Geometry: see drawing. Coordinates: mm, zero at the bounding-box minimum. Coordinates: 2 decimals unless noted, no trailing zeros. Loops run counter-clockwise (first coordinate to the right, second up) from the corner with the lowest first, then second, coordinate; pieces in that order, holes last. Notation, with made-up numbers: (80, 57.5) - (93, 57.5) arc R32 ccw to (93, 83.5) - close; hole circle Ø7 at (-32.5, 49). An arc over 180 degrees is marked (long way). Use a Markdown table: item, result. Add a question column.
1. Section query B-B on z = 2.5. Return the cut outline in (x, y).
2. Ray query, L1, parallel to X at y = 15, z = 3.45; L2, parallel to Z at x = 21, y = 2; L3, parallel to Y at x = 37.5, z = 0.5. Return the intervals inside material, ascending. Write a range as [from, to].
3. Section query D-D on z = 12. Return the cut outline in (x, y).
4. Contact query for flat-ended pins moving along their axis: P1, Ø4, axis at x = 33, y = 19.5, coming from the +Z side; P2, Ø10.5, axis at x = 23.6, y = 15, coming from the -Z side; P3, Ø2, axis at y = 5, z = 2, coming from the -X side; P4, Ø1.5, axis at y = 24, z = 11.5, coming from the +X side. Output: stop coordinate, or through.
5. Draft query along Y for the marked faces 1, 2, 3 and 4. Return one class per face: released by +Y, released by -Y, zero draft, split by the parting line, or undercut.
6. Section query C-C on y = 20.75. Return the cut outline in (x, z).
7. Section query A-A on y = 15. Return the cut outline in (x, z), then the cut area to 3 significant figures.
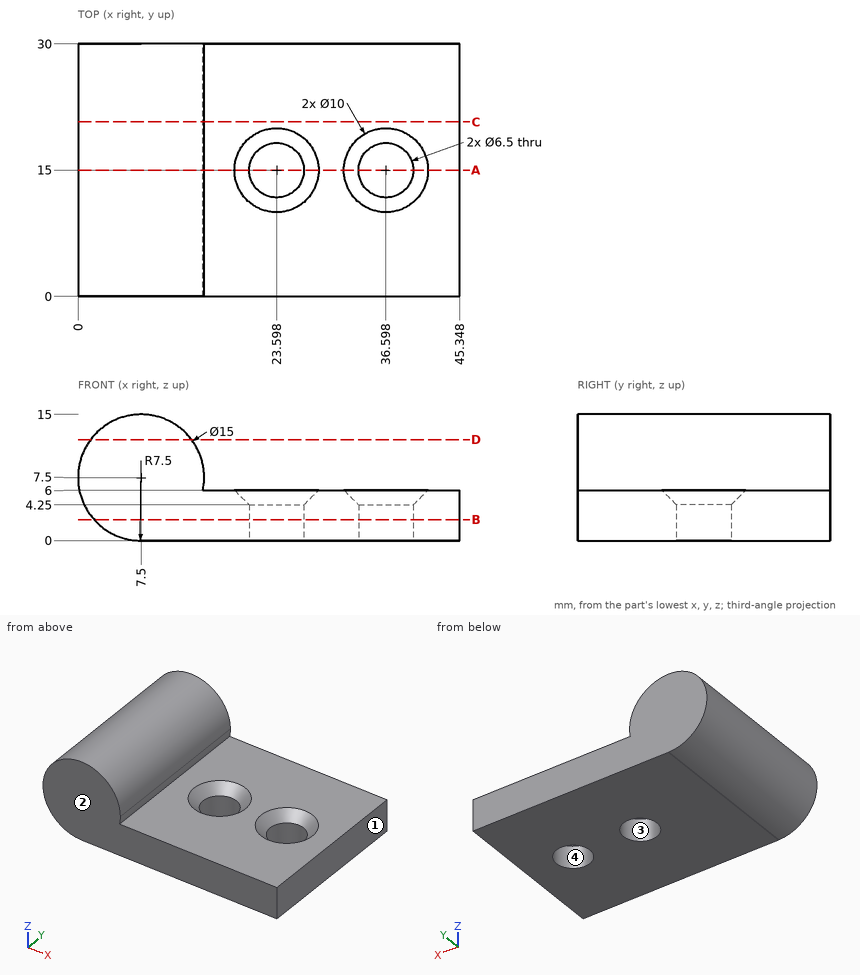
Resolved:
| question | item | result |
|---|---|---|
| 1 | outline | (1.91, 0) - (45.35, 0) - (45.35, 30) - (1.91, 30) - close; hole circle Ø6.5 at (23.6, 15); hole circle Ø6.5 at (36.6, 15) |
| 2 | L1 | [1.19, 20.35], [26.85, 33.35], [39.85, 45.35] |
| 2 | L2 | [0, 6] |
| 2 | L3 | [0, 11.88], [18.12, 30] |
| 3 | outline | (1.5, 0) - (13.5, 0) - (13.5, 30) - (1.5, 30) - close |
| 4 | P1 | z = 6 |
| 4 | P2 | z = 0 |
| 4 | P3 | x = 1.5 |
| 4 | P4 | x = 14.26 |
| 5 | face 1 | zero draft |
| 5 | face 2 | released by -Y |
| 5 | face 3 | undercut |
| 5 | face 4 | undercut |
| 6 | outline | (7.35, 0) arc R7.5 ccw to (7.5, 0) - (45.35, 0) - (45.35, 6) - (14.85, 6) arc R7.5 ccw (long way) to start |
| 7 | outline | (7.35, 0) arc R7.5 ccw to (7.5, 0) - (20.35, 0) - (20.35, 4.25) - (18.6, 6) - (14.85, 6) arc R7.5 ccw (long way) to start; (26.85, 0) - (33.35, 0) - (33.35, 4.25) - (31.6, 6) - (28.6, 6) - (26.85, 4.25) - close; (39.85, 0) - (45.35, 0) - (45.35, 6) - (41.6, 6) - (39.85, 4.25) - close |
| 7 | area | 287 mm² |
